Design review of the part shown in the three views and the two pictorial views. Dimensions are in mm from the part's minimum x, y and z. A direction names the side the tool comes from. Coordinates: 2 decimals unless noted, no trailing zeros. Loops run counter-clockwise (first coordinate to the right, second up) from the corner with the lowest first, then second, coordinate; pieces in that order, holes last. Notation, with made-up numbers: (37.25, 22.25) -> (76.25, 22.25) arc R18 cw to (76.25, 51.25) -> close; hole circle Ø2 at (1.5, 28.5). An arc over 180 degrees is marked (long way). Use a Markdown table: item, result. Add a question column.
Q1. For the marked faces 1 and 2, list the 3-axis set-ups (+Z, -Z, +X, -X, +Y, -Y) from which the entire face can be reached by the end or side of a thin tool; tool diameter is ignored.
Q2. Clearance check with flat-ended pins moving along their axes: pin 1 Ø5 at (y, z) = (48.5, 44.5) entering from -X; pin 2 Ø4 at (x, z) = (45.5, 19.5) entering from -Y; pin 3 Ø14.5 at (x, y) = (63.5, 12.7) entering from -Z; pin 4 Ø2 at (y, z) = (28, 36) entering from +X. State where each tip first meets the part, or that it passes through.
Q3. Draft analysis for pull direction Y (two halves, no side actions). For the marked faces 3, 4, 5 and 6, state which applies: pulls with the +Y half, pulls with the -Y half, needs draft (parallel to the pull), parting line crosses it, or undercut.
Q4. Take a section at D-D on x = 38.1. Write out the cut boundary in (y, z).
Q5. For probe 1 along X at (y, z) = (63, 50); probe 2 along Y at (x, z) = (63.5, 52); probe 3 along Z at (x, y) = (64, 21), list the stretches that pass through material, from the lowest coordinate up.
Q6. Take a section at B-B on z = 47.5. Write out the cut boundary in (x, y).
Q7. Take a section at A-A on x = 12.7. Write out the cut boundary in (y, z).
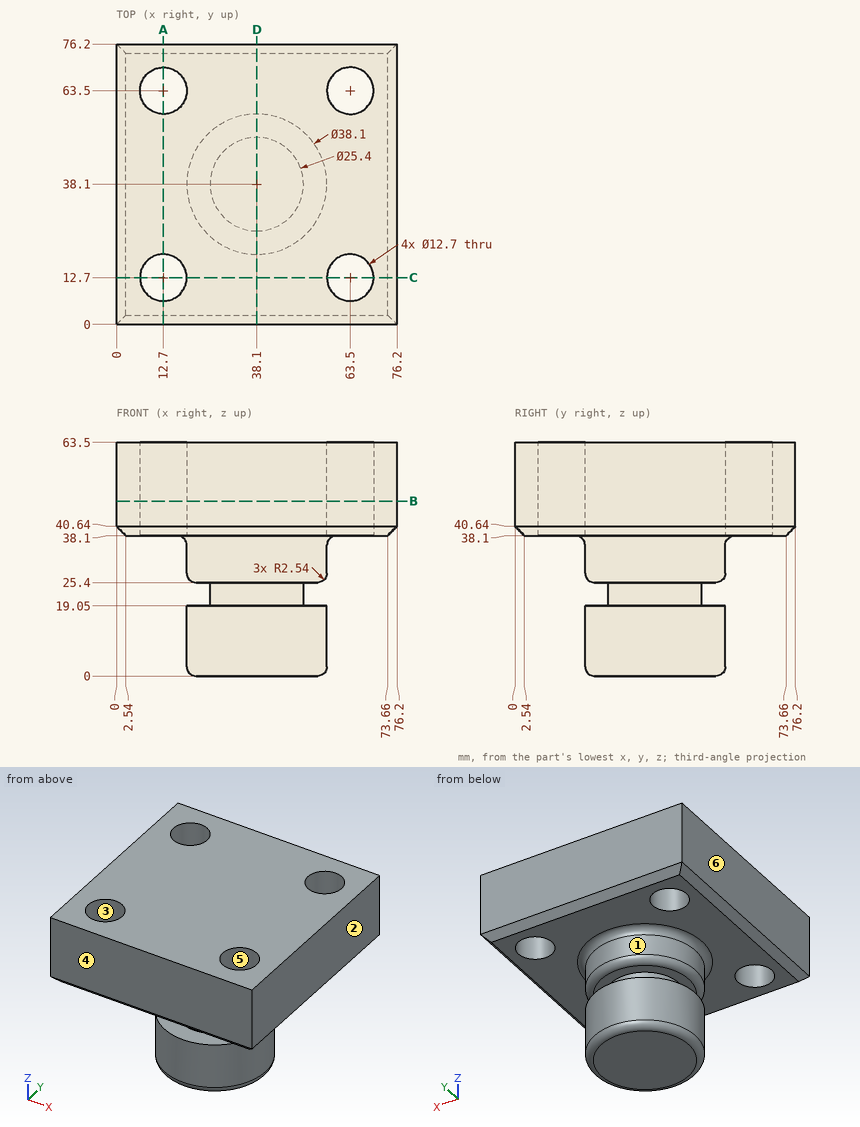
Answer list:
| question | item | result |
|---|---|---|
| 1 | face 1 | -Z |
| 1 | face 2 | +Z, -Z, +X, +Y, -Y |
| 2 | pin 1 | x = 0 |
| 2 | pin 2 | y = 19.85 |
| 2 | pin 3 | z = 38.1 |
| 2 | pin 4 | x = 54.99 |
| 3 | face 3 | undercut |
| 3 | face 4 | pulls with the -Y half |
| 3 | face 5 | undercut |
| 3 | face 6 | needs draft |
| 4 | outline | (0, 40.64) -> (2.54, 38.1) -> (16.51, 38.1) arc R2.54 cw to (19.05, 35.56) -> (19.05, 27.94) arc R2.54 ccw to (21.59, 25.4) -> (25.4, 25.4) -> (25.4, 19.05) -> (19.05, 19.05) -> (19.05, 2.54) arc R2.54 ccw to (21.59, 0) -> (54.61, 0) arc R2.54 ccw to (57.15, 2.54) -> (57.15, 19.05) -> (50.8, 19.05) -> (50.8, 25.4) -> (54.61, 25.4) arc R2.54 ccw to (57.15, 27.94) -> (57.15, 35.56) arc R2.54 cw to (59.69, 38.1) -> (73.66, 38.1) -> (76.2, 40.64) -> (76.2, 63.5) -> (0, 63.5) -> close |
| 5 | probe 1 | 0 to 6.37, 19.03 to 57.17, 69.83 to 76.2 |
| 5 | probe 2 | 0 to 6.35, 19.05 to 57.15, 69.85 to 76.2 |
| 5 | probe 3 | 38.1 to 63.5 |
| 6 | outline | (0, 0) -> (76.2, 0) -> (76.2, 76.2) -> (0, 76.2) -> close; hole circle Ø12.7 at (12.7, 12.7); hole circle Ø12.7 at (12.7, 63.5); hole circle Ø12.7 at (63.5, 12.7); hole circle Ø12.7 at (63.5, 63.5) |
| 7 | outline | (0, 40.64) -> (2.54, 38.1) -> (6.35, 38.1) -> (6.35, 63.5) -> (0, 63.5) -> close; (19.05, 38.1) -> (57.15, 38.1) -> (57.15, 63.5) -> (19.05, 63.5) -> close; (69.85, 38.1) -> (73.66, 38.1) -> (76.2, 40.64) -> (76.2, 63.5) -> (69.85, 63.5) -> close |
